Solid Edge part; units mm, degrees
sketch "Sketch1" plane through (0, 0, 0) normal (0, 0, 1) x (1, 0, 0)
  line L0 (-2.7, 0) -> (2.7, 0)
  line L1 (2.7, 0) -> (2.7, 20.75)
  line L2 (2.7, 20.75) -> (2.5617, 20.75)
  arc A0 (-2.5617, 20.75) -> (2.5617, 20.75) centre (0, 21.75) ccw
  line L3 (-2.7, 20.75) -> (-2.5617, 20.75)
  line L4 (-2.7, 0) -> (-2.7, 20.75)
  dimension "D1" = 2.7
  dimension "D2" = 2.7
extrude "Protrusion1" add sketch "Sketch1" along normal mid plane 6
sketch "Sketch2" plane through (0, 0, 0) normal (0, -1, 0) x (1, 0, 0)
  line L0 (-4.5, -0.95) -> (4.5, -0.95)
  line L1 (4.5, -0.95) -> (4.5, 0.95)
  line L2 (4.5, 0.95) -> (-4.5, 0.95)
  line L3 (-4.5, 0.95) -> (-4.5, -0.95)
  dimension "D1" = 4.5
extrude "Extrusionsausprägung_2" add sketch "Sketch2" against normal blind 8
chamfer "Fase_1" distance 0.5 angle 45 2 edges at (0, 0, 3) (0, 0, -3)
The listing builds one solid part. Answer for the finished solid, in the listing's coordinates (mm). A direction names the side the tool comes from. Coordinates: 2 decimals unless noted, no trailing zeros. Write each loop counter-clockwise with the first axis right and the second up, starting at its lowest first coordinate (ties: lowest second). Pieces come first, ordered by that corner, then holes. Notation, with made-up numbers: (32.25, -25.75) - (72.25, -25.75) arc R19 ccw to (72.25, -12.75) - close; hole circle Ø7 at (61, -13.5). An arc over 180 degrees is marked (long way). Return JSON: item names as keys, results as strings. Group by question number.
Q1. The part is cut by section B-B on y = 7. Write down the section's boundary in (x, z), and give its area (3 significant figures).
Q2. The part is cut by section A-A on z = 0. Write down the section's boundary in (x, y).
Q3. Which of the six approach directions +Z, -Z, +X, -X, +Y, -Y give full straight-line access (tool end or side, diameter ignored) to faces 1 (the flat face through (-4, 4, -0.95)), 2 (the flat face through (4, 4, 0.95)), 3 (the flat face through (-4, 8, 0)), 4 (the flat face through (4, 8, 0))?
Q4. For a pull along X with two mould halves and no side action, classify faces 5 (the flat face through (-4.5, 4, 0)), 6 (the flat face through (-4, 4, 0.95)), 7 (the cylindrical face through (0, 19, 0)) as +X half, -X half, draft (parallel to the pull), parting line (faces both ways), or undercut.
Q5. Find the intervals of material crossed by line 1 along X through (y, z) = (13.75, -0.4); line 2 along Y through (x, z) = (-4, -0.25); line 3 along Y through (x, z) = (0.5, -0.3), in increasing order. Write a range as [from, to].
Q6. The part is cut by section C-C on x = 4. Write down the section's boundary in (y, z), and give its area (3 significant figures).
Q7. The part is cut by section D-D on y = 15.25. Write down the section's boundary in (x, z).
Q8. Flat-ended cylindrical pins translate along their axes: pin 1 Ø0.5 at (x, y) = (3.5, 5.5) entering from +Z; pin 2 Ø0.5 at (x, z) = (-3.5, 0) entering from +Y; pin 3 Ø2 at (x, y) = (-3, 2.5) entering from -Z; pin 4 Ø2 at (x, z) = (0.5, 1) entering from +Y. Find the tip coordinate at first contact, or state that the pin passes through.
Evaluation:
{
 "1": {"outline": "(-4.5, -0.95) - (-2.7, -0.95) - (-2.7, -3) - (2.7, -3) - (2.7, -0.95) - (4.5, -0.95) - (4.5, 0.95) - (2.7, 0.95) - (2.7, 3) - (-2.7, 3) - (-2.7, 0.95) - (-4.5, 0.95) - close", "area": "39.2 mm2"},
 "2": {"outline": "(-4.5, 0) - (4.5, 0) - (4.5, 8) - (2.7, 8) - (2.7, 20.75) - (2.56, 20.75) arc R2.75 cw to (-2.56, 20.75) - (-2.7, 20.75) - (-2.7, 8) - (-4.5, 8) - close"},
 "3": {"face 1": "-Z, -X, +Y, -Y", "face 2": "+Z, +X, +Y, -Y", "face 3": "+Z, -Z, -X, +Y", "face 4": "+Z, -Z, +X, +Y"},
 "4": {"face 5": "-X half", "face 6": "draft", "face 7": "undercut"},
 "5": {"line 1": "x = [-2.7, 2.7]", "line 2": "y = [0, 8]", "line 3": "y = [0, 19.05]"},
 "6": {"outline": "(0, -0.95) - (8, -0.95) - (8, 0.95) - (0, 0.95) - close", "area": "15.2 mm2"},
 "7": {"outline": "(-2.7, -3) - (2.7, -3) - (2.7, 3) - (-2.7, 3) - close"},
 "8": {"pin 1": "stops at z = 0.95", "pin 2": "stops at y = 8", "pin 3": "stops at z = -3", "pin 4": "stops at y = 19.45"}
}
